Could you check a few things on this model? Use its own coordinates, in mm. Coordinates: 2 decimals unless noted, no trailing zeros. Write each loop counter-clockwise with the first axis right and the second up, starting at its lowest first coordinate (ties: lowest second). Pieces come first, ordered by that corner, then holes. Notation, with made-up numbers: M 56.5,47 L 63.5,47 A15 cw 63.5,55 Z; hole C -19.75,72 d4. An arc over 180 degrees is marked long. Answer as CSV lines item,"result". Start each with the question number.
Item 1: If I drill on line 1 along X through (y, z) = (1.95, -11.5); line 2 along X through (y, z) = (4.6, -4.5); line 3 along Z through (x, y) = (30, 1.05), over which ranges is the centre line in solid material (lowest first)? Write a range as [from, to].
Item 2: Suppose I cut it at B-B, the plane y = 0.85. Write out the boundary of the cut face in (x, z).
Item 3: Suppose I cut it at A-A, the plane z = -6.5. Write out the boundary of the cut face in (x, y).
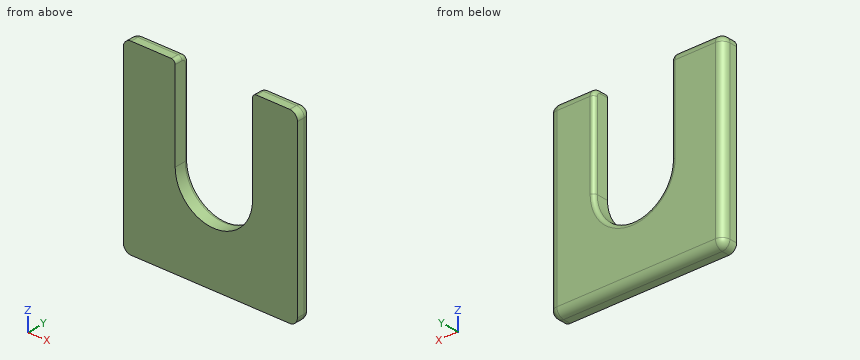
```python
from build123d import *

# Parameters (mm, degrees)
SKETCH1_W           = 57.15
SKETCH1_H           = 60.96
BOSS_EXTRUDE1_DEPTH = 5.08
FILLET1_R           = 2.54
CUT_EXTRUDE1_REACH  = 85.714
FILLET2_R           = 1.27


with BuildPart() as part:
    # Sketch1 → Boss-Extrude1 (new body)
    with BuildSketch(Plane(origin=(0, 0, 0), x_dir=(1, 0, 0), z_dir=(0, 1, 0))):
        with Locations((28.575, 30.48)):
            Rectangle(SKETCH1_W, SKETCH1_H)
    extrude(amount=BOSS_EXTRUDE1_DEPTH)

    # Fillet1
    fillet1_edges = [part.edges().sort_by_distance(p)[0] for p in [
        (57.15, 5.08, -30.48),
        (28.575, 5.08, -60.96),
        (0, 5.08, -30.48),
        (0, 2.54, -60.96),
        (57.15, 2.54, -60.96),
        (57.15, 2.54, 0),
        (0, 2.54, 0),
        (28.575, 5.08, 0),
    ]]
    fillet(fillet1_edges, radius=FILLET1_R)

    # Cut-Extrude1: up to this face of the body (flat: up to its plane)
    cut_extrude1_end = Plane(part.part.faces().sort_by_distance((28.575, 0, -30.48))[0])
    # Sketch2 → Cut-Extrude1 (cut, up to the picked face)
    with BuildSketch(Plane(origin=(0, 5.08, 0), x_dir=(1, 0, 0), z_dir=(0, 1, 0)), mode=Mode.PRIVATE) as cut_extrude1_sk1:
        with BuildLine():
            Line((17.018, 30.48), (17.018, 0))
            Line((17.018, 0), (42.418, 0))
            Line((42.418, 0), (42.418, 30.48))
            ThreePointArc((42.418, 30.48), (29.718, 43.18), (17.018, 30.48))
        make_face()
    cut_extrude1_tool1 = split(extrude(cut_extrude1_sk1.sketch, amount=-CUT_EXTRUDE1_REACH, mode=Mode.PRIVATE), bisect_by=cut_extrude1_end, keep=Keep.BOTH, mode=Mode.PRIVATE)
    add(cut_extrude1_tool1.solids().sort_by(Axis((29.718, 5.08, -20.326586), (0, -1, 0)))[0], mode=Mode.SUBTRACT)

    # Fillet2
    fillet2_edges = [part.edges().sort_by_distance(p)[0] for p in [
        (42.418, 4.336051224, -0.743948776),
        (17.018, 4.336051224, -0.743948776),
        (42.418, 1.27, 0),
        (42.418, 5.08, -16.51),
        (29.718, 5.08, -43.18),
        (17.018, 5.08, -16.51),
        (17.018, 1.27, 0),
    ]]
    fillet(fillet2_edges, radius=FILLET2_R)


solid = part.part
```
Ans:
1,line 1,"x = [0, 17.02], [42.42, 57.15]"
1,line 2,"x = [1.05, 16.74], [42.69, 56.1]"
1,line 3,"z = [-60.96, -43.18]"
2,outline,"M 0,-58.42 A2.54 ccw 2.54,-60.96 L 54.61,-60.96 A2.54 ccw 57.15,-58.42 L 57.15,-2.54 A2.54 ccw 54.61,0 L 43.69,0 A1.27 ccw 42.42,-1.27 L 42.42,-30.48 A12.7 cw 17.02,-30.48 L 17.02,-1.27 A1.27 ccw 15.75,0 L 2.54,0 A2.54 ccw 0,-2.54 Z"
3,outline,"M 0,0 L 17.02,0 L 17.02,3.81 A1.27 ccw 15.75,5.08 L 2.54,5.08 A2.54 ccw 0,2.54 Z; M 42.42,0 L 57.15,0 L 57.15,2.54 A2.54 ccw 54.61,5.08 L 43.69,5.08 A1.27 ccw 42.42,3.81 Z"
